from build123d import *

# Parameters (mm, degrees)
SKETCH1_W               = 355.6
SKETCH1_H               = 76.2
BOSS_EXTRUDE1_DEPTH     = 12.7
CUT_EXTRUDE1_DEPTH      = 183.279291199
CUT_EXTRUDE1_DEPTH_BACK = 183.279291199
SKETCH3_W               = 76.2
SKETCH3_H               = 6.35
BOSS_EXTRUDE2_DEPTH     = 12.7
SKETCH4_W               = 12.7
SKETCH4_H               = 25.4
CUT_EXTRUDE2_DEPTH      = 184.711546997
SKETCH5_R               = 7
CUT_EXTRUDE3_DEPTH      = 184.711546997
CUT_EXTRUDE4_DEPTH      = 184.711546997


with BuildPart() as part:
    # Sketch1 → Boss-Extrude1 (new body)
    with BuildSketch(Plane(origin=(0, 0, 0), x_dir=(0, 0, -1), z_dir=(1, 0, 0))):
        Rectangle(SKETCH1_W, SKETCH1_H)
    extrude(amount=BOSS_EXTRUDE1_DEPTH)

    # Sketch2 → Cut-Extrude1 (cut, two sides: drawn at the far end of the back side and taken through both)
    with BuildSketch(Plane(origin=(12.7, 0, 0), x_dir=(0, 0, -1), z_dir=(1, 0, 0)).offset(-CUT_EXTRUDE1_DEPTH_BACK)):
        Polygon((-507.550847217, -697.601694433), (-177.8, -38.1), (-139.7, 38.1), (190.050847217, 697.601694433), (-1128.95254165, 1357.103388866), (-1826.554236083, -38.1), align=None)
    extrude(amount=CUT_EXTRUDE1_DEPTH + CUT_EXTRUDE1_DEPTH_BACK, mode=Mode.SUBTRACT)

    # Sketch3 → Boss-Extrude2 (add)
    with BuildSketch(Plane.ZY):
        with Locations((-102.87, -41.275)):
            Rectangle(SKETCH3_W, SKETCH3_H)
        with Locations((76.2, -41.275)):
            Rectangle(SKETCH3_W, SKETCH3_H)
        with Locations((-102.87, 41.275)):
            Rectangle(SKETCH3_W, SKETCH3_H)
        with Locations((76.2, 41.275)):
            Rectangle(SKETCH3_W, SKETCH3_H)
    extrude(amount=-BOSS_EXTRUDE2_DEPTH)

    # Sketch4 → Cut-Extrude2 (cut, through all)
    with BuildSketch(Plane.ZY):
        with Locations((-171.45, 0)):
            Rectangle(SKETCH4_W, SKETCH4_H)
    extrude(amount=-CUT_EXTRUDE2_DEPTH, mode=Mode.SUBTRACT)

    # Sketch5 → Cut-Extrude3 (cut, through all)
    with BuildSketch(Plane.ZY):
        with Locations((-102.87, 0)):
            Circle(SKETCH5_R)
    extrude(amount=-CUT_EXTRUDE3_DEPTH, mode=Mode.SUBTRACT)

    # Sketch6 → Cut-Extrude4 (cut, through all)
    with BuildSketch(Plane.ZY):
        Polygon((-13.335, -7.08207294), (-50.428802297, -25.4), (23.758802297, -25.4), align=None)
        Polygon((-27.676197703, 0), (-64.77, 18.31792706), (-64.77, -18.31792706), align=None)
        Polygon((23.758802297, 25.4), (-50.428802297, 25.4), (-13.335, 7.08207294), align=None)
        Polygon((38.1, -18.31792706), (38.1, 18.31792706), (1.006197703, 0), align=None)
        Polygon((105.319743879, -31.75), (82.55, -8.980256121), (59.780256121, -31.75), align=None)
        Polygon((114.3, 22.769743879), (91.530256121, 0), (114.3, -22.769743879), align=None)
        Polygon((73.569743879, 0), (50.8, 22.769743879), (50.8, -22.769743879), align=None)
        Polygon((105.319743879, 31.75), (59.780256121, 31.75), (82.55, 8.980256121), align=None)
    extrude(amount=-CUT_EXTRUDE4_DEPTH, mode=Mode.SUBTRACT)


solid = part.part
Build history of the part. All positions in model axes, mm. A direction names the side the tool comes from. Give positions to 0.01 mm unless a question says otherwise; leave off trailing zeros. Order: outer loops, then holes, each group sorted by start corner. A loop starts at its lowest first (then second) coordinate and runs counter-clockwise, first axis right, second up. Notation, with made-up numbers: M -39.75,70.5 L -13.75,70.5 A29 ccw -13.75,98.5 Z; hole C -21,58.25 d11. An arc over 180 degrees is marked long. Use one line per item in the form item = value.
1) Drop flat-ended pins along their axis: pin 1 (6.5 mm diameter, centred on x = 9, z = -30, fed in from -Y); pin 2 (4 mm diameter, centred on x = 5, z = -32, fed in from +Y); pin 3 (1.9 mm diameter, centred on x = 8.5, y = -42, fed in from -Z); pin 4 (7 mm diameter, centred on x = 9, y = 41.5, fed in from -Z). Give the stop position or say it passes through.
Calculated:
pin_1 = -38.1
pin_2 = 38.1
pin_3 = -140.97
pin_4 = -177.8
2) Probe probe 1 along Y at (x, z) = (2.5, -103); probe 2 along Y at (x, z) = (11.75, 7); probe 3 along Z at (x, y) = (11.25, 3). List the from-to ranges inside material, lowest first.
Calculated:
probe_1 = -44.45 to -7, 7 to 44.45
probe_2 = -38.1 to -25.4, -17.12 to -2.96, 2.96 to 17.12, 25.4 to 38.1
probe_3 = -165.1 to -109.19, -96.55 to -64.77, -33.75 to 7.08, 38.1 to 50.8, 70.57 to 94.53, 114.3 to 157.25
3) Two-plate mould, pull along Z, no slides. Class faces 6 (the face through (6, 38.1, -159)), 7 (the face through (6.3, -16.1, -31.6)): released by +Z, released by -Z, zero draft, split by the parting line, or undercut.
Calculated:
face_6 = zero draft
face_7 = undercut
4) Tool access for faces 1 (the face through (6, 44.45, -103)), 2 (the face through (6, 12.7, -172)), 3 (the face through (6, 38.1, 127)), 4 (the face through (6, -41, 38.1)), 5 (the face through (6.26, -20.21, 71.32)): list every direction of +Z, -Z, +X, -X, +Y, -Y with a clear straight run to the whole face (end or side of a thin tool).
Calculated:
face_1 = +Z, -Z, +X, -X, +Y
face_2 = -Z, +X, -X
face_3 = +Z, +X, -X, +Y
face_4 = +X, -X, -Y
face_5 = +X, -X
5) Saw through at B-B (x = 6). State how many separate pieces and enclosed holes the cut face has, plus the area to 3 significant figures.
Calculated:
separate_pieces = 1
enclosed_holes = 9
area = 22,300 mm2
6) Saw through at A-A (z = -102.87). Give the cut face in (x, y), plus the area to 3 significant figures.
Calculated:
outline = M 0,-44.45 L 12.7,-44.45 L 12.7,-7 L 0,-7 Z; M 0,7 L 12.7,7 L 12.7,44.45 L 0,44.45 Z
area = 951 mm2
7) Saw through at C-C (z = -145). Give the cut face in (x, y), plus the area to 3 significant figures.
Calculated:
outline = M 0,-38.1 L 12.7,-38.1 L 12.7,38.1 L 0,38.1 Z
area = 968 mm2
